Verification items for the finished model (mm, model axes). Face numbers are marked on the shaded views. A direction names the side the tool comes from. Give positions to 0.01 mm unless a question says otherwise; leave off trailing zeros. Order: outer loops, then holes, each group sorted by start corner. A loop starts at its lowest first (then second) coordinate and runs counter-clockwise, first axis right, second up. Notation, with made-up numbers: (-21, 67) -> (31, 67) arc R21 cw to (31, 92) -> close; hole circle Ø7 at (4.5, 52.25). An arc over 180 degrees is marked (long way). Return JSON: item names as keys, results as strings. Group by question number.
(1) Depth check by flat-ended pin: pin 1 Ø17 at (x, y) = (-7.5, 5) entering from +Z; pin 2 Ø12 at (x, z) = (8.5, 39) entering from +Y; pin 3 Ø2.5 at (x, z) = (-0.5, 84.5) entering from +Y. Enter the tip coordinate at first touch or a pass-through.
(2) Tool access check on the marked faces 1 and 2. Record the directions out of +Z, -Z, +X, -X, +Y, -Y that give a thin tool (end or side, any length) a straight path to the whole face; none if there is none.
(3) Cross-section at D-D on x = -4. Enter the section's corners in (y, z).
(4) Thickness scan on line 1 along Z through (x, y) = (-13.5, 9.5); line 2 along Y through (x, z) = (-14, 35); line 3 along Y through (x, z) = (-3, 66). Record the ranges inside material, lowest first.
(5) Cross-section at C-C on z = 58. Enter the section's corners in (x, y), then the cut area to 3 significant figures.
(6) Cross-section at B-B on y = -7. Enter the section's corners in (x, z).
(7) Cross-section at A-A on x = 0. Enter the section's corners in (y, z), then the cut area to 3 significant figures.
from build123d import *

# Parameters (mm, degrees)
SKETCH_1_R          = 17.25
EXTRUDE_1_DEPTH     = 71
SKETCH_2_R          = 6
EXTRUDE_2_DEPTH     = 6
SKETCH_3_R          = 3
EXTRUDE_3_DEPTH     = 15
CUT_EXTRUDE_1_DEPTH = 12


with BuildPart() as part:
    # 草图1 → 凸台-拉伸1 (new body)
    with BuildSketch(Plane.XY):
        Circle(SKETCH_1_R)
    extrude(amount=EXTRUDE_1_DEPTH)

    # 草图2 → 凸台-拉伸2 (add)
    with BuildSketch(Plane.XY.offset(71)):
        with Locations((0, -7)):
            Circle(SKETCH_2_R)
    extrude(amount=EXTRUDE_2_DEPTH)

    # 草图3 → 凸台-拉伸3 (add)
    with BuildSketch(Plane.XY.offset(77)):
        with Locations((0, -7)):
            Circle(SKETCH_3_R)
    extrude(amount=EXTRUDE_3_DEPTH)

    # 草图4 → 切除-拉伸1 (cut)
    with BuildSketch(Plane.XY.offset(92)):
        Polygon((-3.407266726, -4.5), (4.657639837, -4.5), (3.969934626, -3.172821768), (-3.407266726, -3.172821768), align=None)
    extrude(amount=-CUT_EXTRUDE_1_DEPTH, mode=Mode.SUBTRACT)


solid = part.part
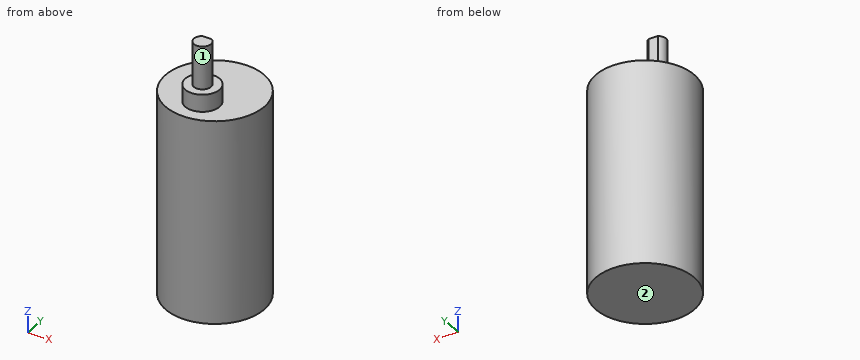
Verdict:
{
 "1": {"pin 1": "z = 77", "pin 2": "y = 17.07", "pin 3": "y = -4.5"},
 "2": {"face 1": "+Z", "face 2": "-Z, +X, -X, +Y, -Y"},
 "3": {"outline": "(-16.78, 0) -> (16.78, 0) -> (16.78, 71) -> (-2.53, 71) -> (-2.53, 77) -> (-11.47, 77) -> (-11.47, 71) -> (-16.78, 71) -> close"},
 "4": {"line 1": "0 to 71", "line 2": "-10.08 to 10.08", "line 3": "-16.99 to 16.99"},
 "5": {"outline": "circle Ø34.5 at (0, 0)", "area": "935 mm²"},
 "6": {"outline": "(-15.77, 0) -> (15.77, 0) -> (15.77, 71) -> (6, 71) -> (6, 77) -> (3, 77) -> (3, 92) -> (-3, 92) -> (-3, 77) -> (-6, 77) -> (-6, 71) -> (-15.77, 71) -> close"},
 "7": {"outline": "(-17.25, 0) -> (17.25, 0) -> (17.25, 71) -> (-1, 71) -> (-1, 77) -> (-4, 77) -> (-4, 80) -> (-4.5, 80) -> (-4.5, 92) -> (-10, 92) -> (-10, 77) -> (-13, 77) -> (-13, 71) -> (-17.25, 71) -> close", "area": "2,610 mm²"}
}
